Check sheet for the drawn part. Datum: minimum x, y, z corner. Units: mm. A direction names the side the tool comes from. Coordinates: 2 decimals unless noted, no trailing zeros. Order: outer loops, then holes, each group sorted by start corner. A loop starts at its lowest first (then second) coordinate and runs counter-clockwise, first axis right, second up. Notation, with made-up numbers: (35.25, 26) - (46.25, 26) arc R24 cw to (46.25, 60) - close; hole circle Ø5 at (75.25, -10). An arc over 180 degrees is marked (long way). One line per item, written item: value. Start each with the question number.
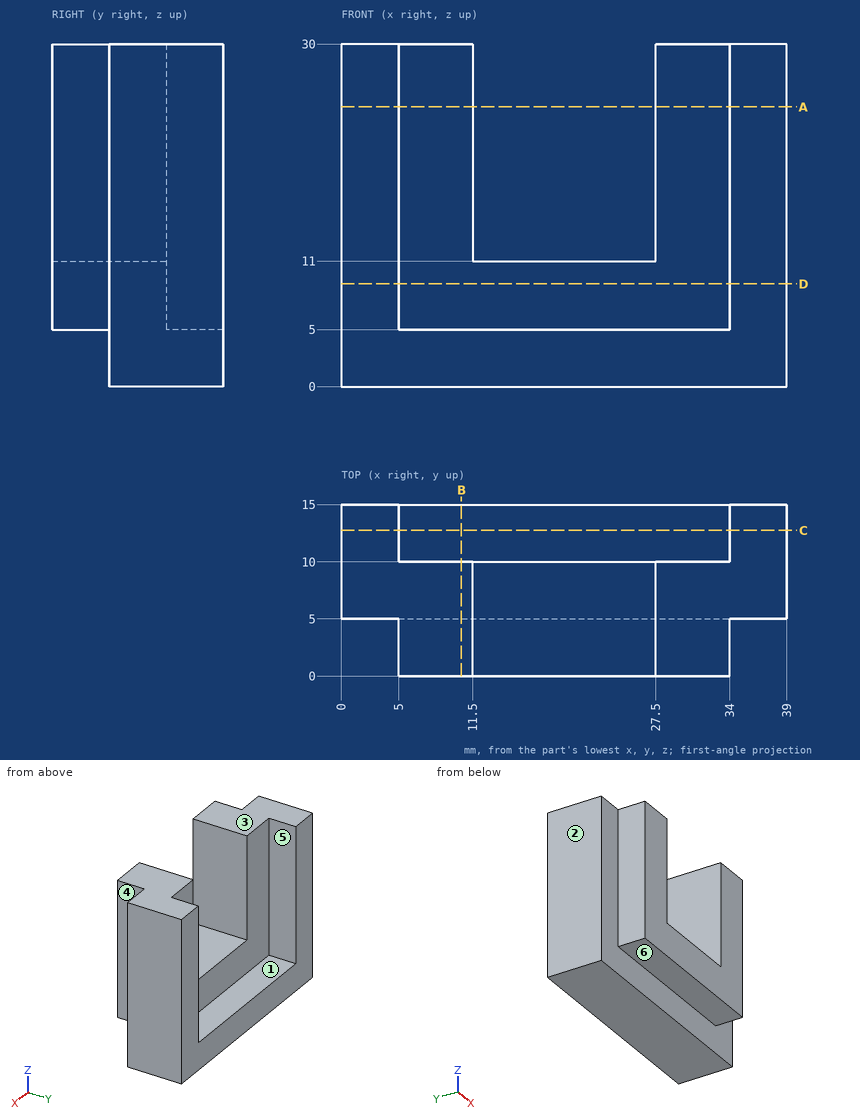
Q1. Material ranges on probe 1 along X at (y, z) = (9, 24.75); probe 2 along X at (y, z) = (1.25, 28); probe 3 along Z at (x, y) = (18.5, 4.5), recorded low to high.
Q2. Gauge pin test, flat ends, axial feed: P1, Ø3, axis at x = 21, y = 13, coming from the +Z side; P2, Ø2, axis at y = 3, z = 12.5, coming from the +X side; P3, Ø9, axis at x = 22.5, z = 16.5, coming from the -Y side; P4, Ø5.5, axis at x = 17.5, y = 2, coming from the -Z side. Record the tip position at first contact, or that the pin passes through.
Q3. Cross-section at A-A, the plane z = 24.5. Enter the section's corners in (x, y).
Q4. Set-up check for the marked faces 4, 5 and 6: record each of +Z, -Z, +X, -X, +Y, -Y from which the full face is reachable in a straight line by a thin tool's end or side.
Q5. Cross-section at B-B, the plane x = 10.5. Enter the section's corners in (y, z), and give its area (3 significant figures).
Q6. Cross-section at D-D, the plane z = 9. Enter the section's corners in (x, y).
Q7. Cross-section at C-C, the plane y = 12.75. Enter the section's corners in (x, z), and give its area (3 significant figures).
Q8. Release check for a two-part mould opening along X. For the marked faces 1, 2 and 3 record: released by +X, released by -X, zero draft, split by the parting line, or undercut.
Check result:
1. probe 1: x = 0 to 11.5, 27.5 to 39
1. probe 2: x = 5 to 11.5, 27.5 to 34
1. probe 3: z = 5 to 11
2. P1: stops at z = 5
2. P2: stops at x = 34
2. P3: passes through
2. P4: stops at z = 5
3. outline: (0, 5) - (5, 5) - (5, 0) - (11.5, 0) - (11.5, 10) - (5, 10) - (5, 15) - (0, 15) - close; (27.5, 0) - (34, 0) - (34, 5) - (39, 5) - (39, 15) - (34, 15) - (34, 10) - (27.5, 10) - close
4. face 4: +Z, -Z, +X, -Y
4. face 5: +Z, +Y
4. face 6: -Z, +X, -X, -Y
5. outline: (0, 5) - (5, 5) - (5, 0) - (15, 0) - (15, 5) - (10, 5) - (10, 30) - (0, 30) - close
5. area: 300 mm2
6. outline: (0, 5) - (5, 5) - (5, 0) - (34, 0) - (34, 5) - (39, 5) - (39, 15) - (34, 15) - (34, 10) - (5, 10) - (5, 15) - (0, 15) - close
7. outline: (0, 0) - (39, 0) - (39, 30) - (34, 30) - (34, 5) - (5, 5) - (5, 30) - (0, 30) - close
7. area: 445 mm2
8. face 1: undercut
8. face 2: released by -X
8. face 3: zero draft
